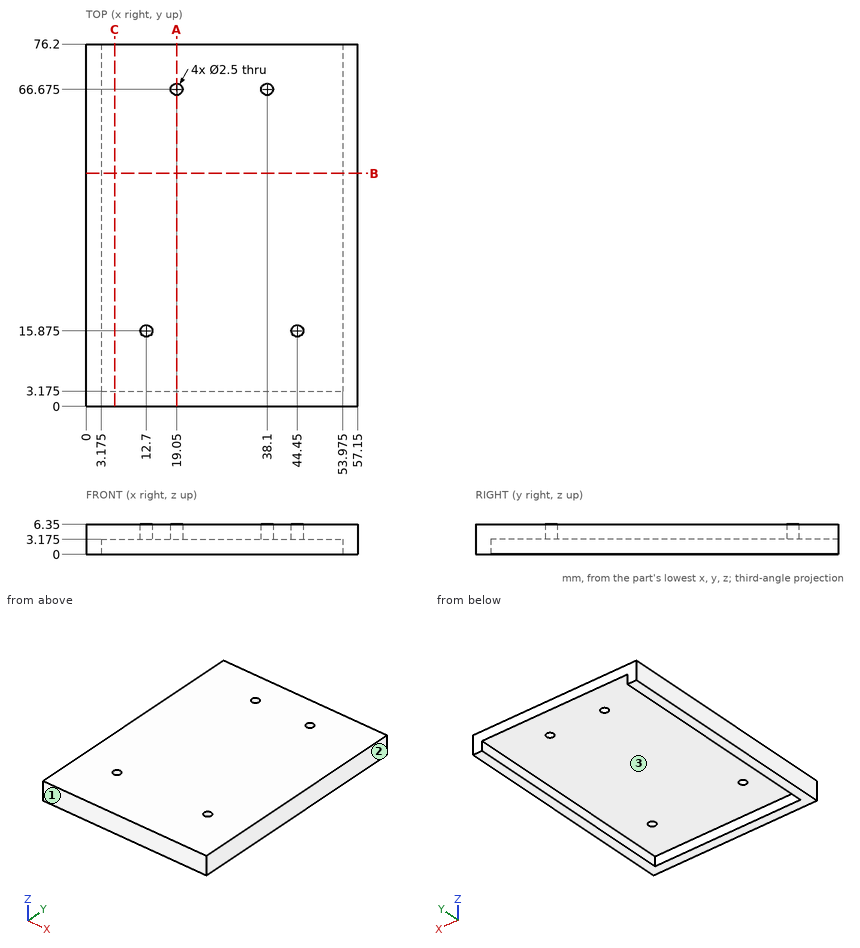
Part print with two shaded views. Sizes in mm from the minimum x, y, z corner. Coordinates: 2 decimals unless noted, no trailing zeros. Write each loop counter-clockwise with the first axis right and the second up, starting at its lowest first coordinate (ties: lowest second). Pieces come first, ordered by that corner, then holes.
1. Band-saw the part on B-B, the plane y = 49. Give the cut face in (x, z) (3 decimals), and give its area (3 significant figures).
Answer block:
outline: (0, 0) - (3.175, 0) - (3.175, 3.175) - (53.975, 3.175) - (53.975, 0) - (57.15, 0) - (57.15, 6.35) - (0, 6.35) - close
area: 202 mm2
2. Band-saw the part on C-C, the plane x = 6. Give the cut face in (y, z) (3 decimals), and give its area (3 significant figures).
Answer block:
outline: (0, 0) - (3.175, 0) - (3.175, 3.175) - (76.2, 3.175) - (76.2, 6.35) - (0, 6.35) - close
area: 252 mm2
3. Drill centre lines: probe 1 along Y at (x, z) = (12.7, 4) (3 decimals); probe 2 along Y at (x, z) = (38, 3.75); probe 3 along X at (y, z) = (31.5, 0.5) (3 decimals). Where is each one in solid material? Low to high.
Answer block:
probe 1: y = 0 to 14.625, 17.125 to 76.2
probe 2: y = 0 to 65.43, 67.92 to 76.2
probe 3: x = 0 to 3.175, 53.975 to 57.15
4. Band-saw the part on A-A, the plane x = 19.05. Give the cut face in (y, z) (3 decimals).
Answer block:
outline: (0, 0) - (3.175, 0) - (3.175, 3.175) - (65.425, 3.175) - (65.425, 6.35) - (0, 6.35) - close; (67.925, 3.175) - (76.2, 3.175) - (76.2, 6.35) - (67.925, 6.35) - close
5. Drop flat-ended pins along their axis: pin 1 (3 mm diameter, centred on x = 44.45, y = 15.875, fed in from -Z) (3 decimals); pin 2 (1 mm diameter, centred on x = 19.5, z = 1, fed in from +Y) (3 decimals). Give the stop position or say it passes through.
Answer block:
pin 1: stops at z = 3.175
pin 2: stops at y = 3.175
6. Pull direction X, two halves, no side cores. Call the marked faces 1, 2 and 3: released by +X, released by -X, zero draft, split by the parting line, or undercut.
Answer block:
face 1: zero draft
face 2: released by +X
face 3: undercut
